Can you work these out from the model? Positions are in its coordinate system, mm. Give positions to 0.01 mm unless a question says otherwise; leave off trailing zeros. Order: outer loops, then holes, each group sorted by start corner. A loop starts at its lowest first (then second) coordinate and runs counter-clockwise, first axis right, second up. Notation, with made-up numbers: (74, -21) - (91, -21) arc R25 cw to (91, 7) - close; hole circle Ø4 at (-37.5, 84.5). An arc over 180 degrees is marked (long way). Answer as a JSON object with one key per item and string values.
```python
from build123d import *

# Parameters (mm, degrees)
ESBO_O1_W                = 145
ESBO_O1_H                = 260
RESSALTO_EXTRUS_O1_DEPTH = 4
FURO_COM_FOLGA_DE_M41_D  = 4.5
FILETE1_R                = 20


with BuildPart() as part:
    # Esboço1 → Ressalto-extrusão1 (new body)
    with BuildSketch(Plane.XY):
        Rectangle(ESBO_O1_W, ESBO_O1_H)
        with BuildLine():
            Line((-34.5, -95), (34.5, -95))
            ThreePointArc((34.5, -95), (36.621320344, -94.121320344), (37.5, -92))
            Line((37.5, -92), (37.5, 92))
            ThreePointArc((37.5, 92), (36.621320344, 94.121320344), (34.5, 95))
            Line((34.5, 95), (-34.5, 95))
            ThreePointArc((-34.5, 95), (-36.621320344, 94.121320344), (-37.5, 92))
            Line((-37.5, 92), (-37.5, -92))
            ThreePointArc((-37.5, -92), (-36.621320344, -94.121320344), (-34.5, -95))
        make_face(mode=Mode.SUBTRACT)
    extrude(amount=RESSALTO_EXTRUS_O1_DEPTH)

    # Furo com folga de M41 (through all)
    with Locations(Plane.XY.offset(4)):
        with Locations((-37.5, 123), (37.5, 123), (65.5, 55), (65.5, -55), (37.5, -123), (-37.5, -123), (-65.5, -55), (-65.5, 55)):
            Hole(FURO_COM_FOLGA_DE_M41_D / 2)

    # Filete1
    filete1_edges = [part.edges().sort_by_distance(p)[0] for p in [
        (72.5, -130, 2),
        (-72.5, -130, 2),
        (-72.5, 130, 2),
        (72.5, 130, 2),
    ]]
    fillet(filete1_edges, radius=FILETE1_R)


solid = part.part
```
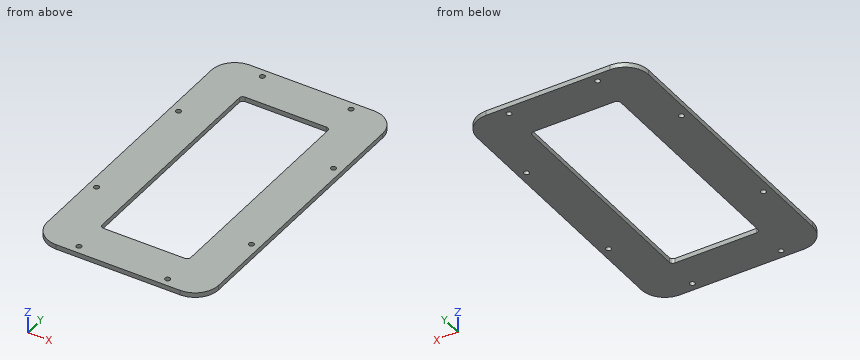
Q1. If we section it at A-A, the plane x = -5.5: Please give me the cut outline in (y, z).
Recorded:
{"outline": "(-130, 0) - (-95, 0) - (-95, 4) - (-130, 4) - close; (95, 0) - (130, 0) - (130, 4) - (95, 4) - close"}
Q2. I need wall thicknesses on L1, parallel to Y at x = -65.5, z = 2.95; L2, parallel to X at y = -54.5, z = 0.5; L3, parallel to Y at x = -9, z = 2.1. Which ranges of each line are inside material? Lowest first, please.
Recorded:
{"L1": "y = -125.2 to -57.25, -52.75 to 52.75, 57.25 to 125.2", "L2": "x = -72.5 to -67.69, -63.31 to -37.5, 37.5 to 63.31, 67.69 to 72.5", "L3": "y = -130 to -95, 95 to 130"}
Q3. If we section it at B-B, the plane y = -75: Please give me the cut outline in (x, z).
Recorded:
{"outline": "(-72.5, 0) - (-37.5, 0) - (-37.5, 4) - (-72.5, 4) - close; (37.5, 0) - (72.5, 0) - (72.5, 4) - (37.5, 4) - close"}
Q4. If we section it at C-C, the plane z = 2.25: Count the separate pieces of the cut face and the enclosed holes in it, then the cut area to 3 significant figures.
Recorded:
{"separate pieces": "1", "enclosed holes": "9", "area": "23,000 mm^2"}
